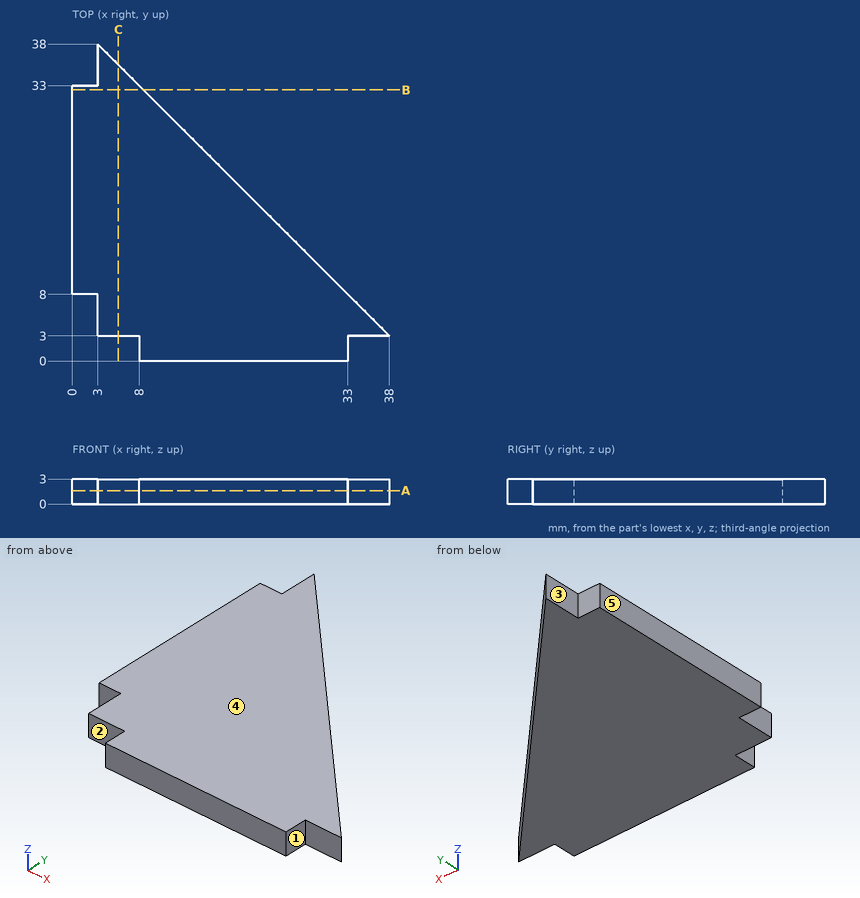
The drawing under review shows one solid part. Ordinate dimensions are in mm from its lowest x, y, z. A direction names the side the tool comes from. Give positions to 0.01 mm unless a question says otherwise; leave off trailing zeros. Order: outer loops, then holes, each group sorted by start corner. A loop starts at its lowest first (then second) coordinate and runs counter-clockwise, first axis right, second up. Notation, with made-up numbers: M 37.25,83.5 L 92.25,83.5 A34 cw 92.25,120.5 Z; hole C -33.75,24 d2. An arc over 180 degrees is marked long. One line per question, with ' | ' between items. Start each with the question number.
Q1. For L1, parallel to Y at x = 2.5, z = 2.35; L2, parallel to Y at x = 32, z = 1.35; L3, parallel to X at y = 11, z = 1.4, list the stretches that pass through material, from the lowest coordinate up. Write a range as [from, to].
Q2. We need section C-C (x = 5.5). Write out the cut boundary in (y, z), plus the area to 3 significant figures.
Q3. We need section A-A (z = 1.6). Write out the cut boundary in (x, y).
Q4. For pin 1 Ø1.5 at (y, z) = (33.5, 0.5) entering from +X; pin 2 Ø0.9 at (y, z) = (1, 1) entering from +X; pin 3 Ø0.9 at (x, z) = (36.5, 1.5) entering from -Y, all flat-tipped, find the tip position at first contact; note any pin that passes through.
Q5. We need section B-B (y = 32.5). Write out the cut boundary in (x, z), plus the area to 3 significant figures.
Q6. Machinability: for the marked faces 1, 2, 3, 4 and 5, which of the approach directions +Z, -Z, +X, -X, +Y, -Y give a long, thin tool a straight path to every point of the face, cutting with its end or side? Answer none if there is none.
Returned:
1) L1: [8, 33] | L2: [0, 9] | L3: [0, 30]
2) outline: M 3,0 L 35.5,0 L 35.5,3 L 3,3 Z | area: 97.5 mm2
3) outline: M 0,8 L 3,8 L 3,3 L 8,3 L 8,0 L 33,0 L 33,3 L 38,3 L 3,38 L 3,33 L 0,33 Z
4) pin 1: x = 8.25 | pin 2: x = 33 | pin 3: y = 3
5) outline: M 0,0 L 8.5,0 L 8.5,3 L 0,3 Z | area: 25.5 mm2
6) face 1: +Z, -Z, +X, -Y | face 2: +Z, -Z, -X, -Y | face 3: +Z, -Z, -X, +Y | face 4: +Z, +X, -X, +Y, -Y | face 5: +Z, -Z, -X, +Y, -Y
